Here's how the part is built. I have some questions about the finished solid (model axes, mm). A direction names the side the tool comes from. Coordinates: 2 decimals unless noted, no trailing zeros. Write each loop counter-clockwise with the first axis right and the second up, starting at its lowest first coordinate (ties: lowest second). Pieces come first, ordered by that corner, then holes.
(1) Imagine slicing it at C-C, the plane y = 25. List the corners of the cut face in (x, z) for me, plus the area to 4 significant figures.
(2) Imagine slicing it at A-A, the plane x = 0. List the corners of the cut face in (y, z) for me.
(3) Please list where these lines run through material, in increasing order: probe 1 along X at (y, z) = (-3, -56); probe 2 along X at (y, z) = (69, 1.5); probe 3 along Z at (x, y) = (-7.5, 34).
(4) Imagine slicing it at B-B, the plane z = -56. List the corners of the cut face in (x, y) for me.
(5) Thinking about a two-plate mould opening in X: for faces 4 (the flat face through (-32.5, 14, -14)), 5 (the cylindrical face through (41.372, 9.209, -9.357)), 6 (the flat face through (-27.5, 14, -14)), 7 (the cylindrical face through (0.385, 9.209, -9.357)), which applies, released by +X, released by -X, zero draft, split by the parting line, or undercut?
(6) Which directions (+Z, -Z, +X, -X, +Y, -Y) give clear straight access to the entire face, cutting with the end or side of a thin tool? Please do faces 1 (the flat face through (32.5, 14, -14)), 2 (the flat face through (0.7, 59.6, 6.5)), 3 (the flat face through (27.5, 14, -14)).
(7) Imagine slicing it at D-D, the plane y = 69. List the corners of the cut face in (x, z) for me, plus the area to 3 significant figures.
(8) For pin 1 Ø6 at (x, y) = (23.5, 75) entering from -Z, with a flat end and sliding along its axis, tell me the tip position at first contact or that it passes through.
```python
from build123d import *

# Parameters (mm, degrees)
ESTRUSIONE_SOTTILE1_DEPTH = 50
SCHIZZO2_R                = 9
TAGLIO_ESTRUSIONE1_DEPTH  = 148.764170217
SCHIZZO3_R                = 6.5
TAGLIO_ESTRUSIONE2_DEPTH  = 148.720174655
NERVATURA1_REACH          = 166.332
SCHIZZO4_WALL_W           = 358.948233372
SCHIZZO4_WALL_H           = 5


with BuildPart() as part:
    # Schizzo1 → Estrusione-Sottile1 (new, symmetric)
    with BuildSketch(Plane(origin=(0, 0, 0), x_dir=(0, 0, -1), z_dir=(1, 0, 0))):
        with BuildLine():
            Line((-6.5, 102), (-6.5, 16))
            ThreePointArc((-6.5, 16), (0.090097423, 0.090097423), (16, -6.5))
            Line((16, -6.5), (101, -6.5))
            Line((101, -6.5), (101, 6.5))
            Line((101, 6.5), (16, 6.5))
            ThreePointArc((16, 6.5), (9.282485579, 9.282485579), (6.5, 16))
            Line((6.5, 16), (6.5, 102))
            Line((6.5, 102), (-6.5, 102))
        make_face()
    extrude(amount=ESTRUSIONE_SOTTILE1_DEPTH, both=True)

    # Schizzo2 → Taglio-Estrusione1 (cut, through all)
    with BuildSketch(Plane(origin=(0, 0, -6.5), x_dir=(-1, 0, 0), z_dir=(0, 0, -1))):
        with Locations(Location((0, 69, 0), (0, 0, 90))):
            Circle(SCHIZZO2_R)
    extrude(amount=-TAGLIO_ESTRUSIONE1_DEPTH, mode=Mode.SUBTRACT)

    # Schizzo3 → Taglio-Estrusione2 (cut, through all)
    with BuildSketch(Plane(origin=(0, 6.5, 0), x_dir=(1, 0, 0), z_dir=(0, 1, 0))):
        with Locations(Location((-23.683594655, 56, 0), (0, 0, 270))):
            Circle(SCHIZZO3_R)
        with Locations(Location((26.316405345, 56, 0), (0, 0, 270))):
            Circle(SCHIZZO3_R)
    extrude(amount=-TAGLIO_ESTRUSIONE2_DEPTH, mode=Mode.SUBTRACT)

    # Schizzo4 wall → Nervatura1 (add, up to next)
    with BuildSketch(Plane(origin=(30, 16.5, -16.5), x_dir=(0, -0.707106781187, -0.707106781187), z_dir=(0, 0.707106781187, -0.707106781187)), mode=Mode.PRIVATE) as nervatura1_sk1:
        Rectangle(SCHIZZO4_WALL_W, SCHIZZO4_WALL_H)
    nervatura1_tool1 = extrude(nervatura1_sk1.sketch, amount=-NERVATURA1_REACH, mode=Mode.PRIVATE) - part.part
    nervatura1 = nervatura1_tool1.solids().sort_by_distance((30, 16.5, -16.5))[0]
    add(nervatura1)

    # Specchia1: Nervatura1 across plane
    add(nervatura1.mirror(Plane(origin=(0, 0, 0), x_dir=(0, 0, 1), z_dir=(1, 0, 0))))


solid = part.part
```
Recorded:
1. outline: (-50, -6.5) - (-32.5, -6.5) - (-32.5, -8) - (-27.5, -8) - (-27.5, -6.5) - (27.5, -6.5) - (27.5, -8) - (32.5, -8) - (32.5, -6.5) - (50, -6.5) - (50, 6.5) - (-50, 6.5) - close
1. area: 1,315 mm2
2. outline: (-6.5, -101) - (6.5, -101) - (6.5, -16) arc R9.5 cw to (16, -6.5) - (60, -6.5) - (60, 6.5) - (16, 6.5) arc R22.5 ccw to (-6.5, -16) - close; (78, -6.5) - (102, -6.5) - (102, 6.5) - (78, 6.5) - close
3. probe 1: x = -50 to -30.18, -17.18 to 19.82, 32.82 to 50
3. probe 2: x = -50 to -9, 9 to 50
3. probe 3: z = -6.5 to 6.5
4. outline: (-50, -6.5) - (-30.18, -6.5) - (-30.18, 6.5) - (-50, 6.5) - close; (-17.18, -6.5) - (19.82, -6.5) - (19.82, 6.5) - (-17.18, 6.5) - close; (32.82, -6.5) - (50, -6.5) - (50, 6.5) - (32.82, 6.5) - close
5. face 4: released by -X
5. face 5: zero draft
5. face 6: undercut
5. face 7: undercut
6. face 1: -Z, +X, +Y
6. face 2: +Z, +X, -X, +Y, -Y
6. face 3: -Z, +Y
7. outline: (-50, -6.5) - (-9, -6.5) - (-9, 6.5) - (-50, 6.5) - close; (9, -6.5) - (50, -6.5) - (50, 6.5) - (9, 6.5) - close
7. area: 1,070 mm2
8. pin 1: stops at z = -6.5
